Source: CAD feature listing. Evaluate the final solid. Frame: model axes, mm. A direction names the side the tool comes from. Coordinates: 2 decimals unless noted, no trailing zeros. Loops run counter-clockwise (first coordinate to the right, second up) from the corner with the lowest first, then second, coordinate; pieces in that order, holes last. Notation, with made-up numbers: (-8, 56) -> (18, 56) arc R14 ccw to (18, 67) -> close; hole circle Ø7 at (64.5, 19). An arc over 180 degrees is marked (long way). Answer as CSV lines item,"result".
from build123d import *

# Parameters (mm, degrees)
SKETCH3_W                           = 101.6
SKETCH3_H                           = 11.1125
BOSS_EXTRUDE1_DEPTH                 = 50.8
BASEBORDERRADIUSSKETCH_OUTSIDE_W    = 132.41
BASEBORDERRADIUSSKETCH_OUTSIDE_H    = 132.41
BASEBORDERRADIUSSKETCH_OUTSIDE_W_2  = 95.25
BASEBORDERRADIUSSKETCH_OUTSIDE_H_2  = 95.25
BASEBORDERRADIUSCUT_EXTRUDE_DEPTH   = 73.57931249
BUMPER_6_32_TAPPED_HOLE_D           = 4.3053
BUMPER_6_32_TAPPED_HOLE_CBORE_D     = 7.9375
BUMPER_6_32_TAPPED_HOLE_CBORE_DEPTH = 5.3848
BUMPERTHREADLPATTERN_COUNT          = 2
BUMPERTHREADLPATTERN_PITCH          = 76.2
BUMPERTHREADLPATTERN_COUNT_DIR2     = 2
BUMPERTHREADLPATTERN_PITCH_DIR2     = 76.2


with BuildPart() as part:
    # Sketch3 → Boss-Extrude1 (new, symmetric)
    with BuildSketch(Plane.XY):
        Rectangle(SKETCH3_W, SKETCH3_H)
    extrude(amount=BOSS_EXTRUDE1_DEPTH, both=True)

    # FacingTopSurfaceCut
    split(bisect_by=Plane(origin=(0, 5.159375, 0), x_dir=(1, 0, 0), z_dir=(0, 1, 0)), keep=Keep.BOTTOM)

    # FacingBottomSurfaceCut
    split(bisect_by=Plane(origin=(0, -5.159375, 0), x_dir=(-1, 0, 0), z_dir=(0, -1, 0)), keep=Keep.BOTTOM)

    # BaseBorderRadiusSketch outside → BaseBorderRadiusCut-Extrude (cut, through all)
    with BuildSketch(Plane(origin=(0, 5.159375, 0), x_dir=(1, 0, 0), z_dir=(0, 1, 0))):
        Rectangle(BASEBORDERRADIUSSKETCH_OUTSIDE_W, BASEBORDERRADIUSSKETCH_OUTSIDE_H)
        Rectangle(BASEBORDERRADIUSSKETCH_OUTSIDE_W_2, BASEBORDERRADIUSSKETCH_OUTSIDE_H_2, mode=Mode.SUBTRACT)
    extrude(amount=-BASEBORDERRADIUSCUT_EXTRUDE_DEPTH, mode=Mode.SUBTRACT)

    # Bumper#6-32 Tapped Hole (through all)
    with Locations(Plane(origin=(-38.1, -5.159375, 38.1), x_dir=(0, 0, -1), z_dir=(0, -1, 0))):
        with Locations((0, 0)):
            bumper_6_32_tapped_hole = CounterBoreHole(BUMPER_6_32_TAPPED_HOLE_D / 2, BUMPER_6_32_TAPPED_HOLE_CBORE_D / 2, BUMPER_6_32_TAPPED_HOLE_CBORE_DEPTH)

    # BumperThreadLPattern: Bumper_6-32 Tapped Hole 2 × 2
    with Locations(*[(j * BUMPERTHREADLPATTERN_PITCH_DIR2, 0, -i * BUMPERTHREADLPATTERN_PITCH) for i in range(BUMPERTHREADLPATTERN_COUNT) for j in range(BUMPERTHREADLPATTERN_COUNT_DIR2) if (i, j) != (0, 0)]):
        add(bumper_6_32_tapped_hole, mode=Mode.SUBTRACT)


solid = part.part
(1) Cut plane B-B (x = -38.1). Return the cut outline in (y, z) (3 decimals), then the cut area to 3 significant figures.
Computed values:
outline,"(-5.159, -47.625) -> (5.159, -47.625) -> (5.159, -40.253) -> (0.225, -40.253) -> (0.225, -42.069) -> (-5.159, -42.069) -> close; (-5.159, -34.131) -> (0.225, -34.131) -> (0.225, -35.947) -> (5.159, -35.947) -> (5.159, 35.947) -> (0.225, 35.947) -> (0.225, 34.131) -> (-5.159, 34.131) -> close; (-5.159, 42.069) -> (0.225, 42.069) -> (0.225, 40.253) -> (5.159, 40.253) -> (5.159, 47.625) -> (-5.159, 47.625) -> close"
area,"855 mm^2"
(2) Cut plane A-A (z = -38.1). Return the cut outline in (x, y) (3 decimals), then the cut area to 3 significant figures.
Computed values:
outline,"(-47.625, -5.159) -> (-42.069, -5.159) -> (-42.069, 0.225) -> (-40.253, 0.225) -> (-40.253, 5.159) -> (-47.625, 5.159) -> close; (-35.947, 0.225) -> (-34.131, 0.225) -> (-34.131, -5.159) -> (34.131, -5.159) -> (34.131, 0.225) -> (35.947, 0.225) -> (35.947, 5.159) -> (-35.947, 5.159) -> close; (40.253, 0.225) -> (42.069, 0.225) -> (42.069, -5.159) -> (47.625, -5.159) -> (47.625, 5.159) -> (40.253, 5.159) -> close"
area,"855 mm^2"
(3) Pin query (flat end, axial travel): pin 1 Ø2.5 at (x, z) = (38.1, 38.1) entering from +Y; pin 2 Ø4 at (x, z) = (-38, -39) entering from -Y. Return the tip coordinate at first contact, or that it passes through.
Computed values:
pin 1,"through"
pin 2,"y = 0.23"
(4) Material intervals for L1, parallel to X at y = 1.7, z = 38.1 (3 decimals); L2, parallel to X at y = -3.9, z = 38.1 (3 decimals); L3, parallel to Z at x = 35, y = -2.5 (3 decimals), sorted ascending. Write a range as [from, to].
Computed values:
L1,"[-47.625, -40.253], [-35.947, 35.947], [40.253, 47.625]"
L2,"[-47.625, -42.069], [-34.131, 34.131], [42.069, 47.625]"
L3,"[-47.625, -40.578], [-35.622, 35.622], [40.578, 47.625]"
(5) Draft query along Z for faces 3 (the flat face through (-1, 0, -47.625)), 4 (the cylindrical face through (-41.62, -2.5, 36.27)), 5 (the flat face through (-47.625, 0, 1)), 6 (the cylindrical face through (40.234, 2.727, 37.82)). Return one class per face: released by +Z, released by -Z, zero draft, split by the parting line, or undercut.
Computed values:
face 3,"released by -Z"
face 4,"undercut"
face 5,"zero draft"
face 6,"undercut"
(6) Access query for faces 1 (the flat face through (47.625, 0, 1)), 2 (the flat face through (36, 0.225, 36)). Directions: +Z, -Z, +X, -X, +Y, -Y. A direction counts if a zero-diameter tool reaches every point of the face in a straight line with its end or side. Return the directions, or none.
Computed values:
face 1,"+Z, -Z, +X, +Y, -Y"
face 2,"-Y"
